Could you check a few things on this model? Use its own coordinates, in mm. A direction names the side the tool comes from. Coordinates: 2 decimals unless noted, no trailing zeros. Write each loop counter-clockwise with the first axis right and the second up, starting at its lowest first coordinate (ties: lowest second). Pieces come first, ordered by that corner, then holes.
```python
from build123d import *

# Parameters (mm, degrees)
SKETCH_1_W          = 95
SKETCH_1_H          = 55
EXTRUDE_1_DEPTH     = 5.5
SKETCH_3_W          = 5.5
SKETCH_3_H          = 20
CUT_EXTRUDE_2_DEPTH = 56.161127617
SKETCH_4_W          = 20
SKETCH_4_H          = 5.504098133
SKETCH_4_W_2        = 5
CUT_EXTRUDE_3_DEPTH = 56.161127617


with BuildPart() as part:
    # ｽｹｯﾁ1 → ﾎﾞｽ - 押し出し1 (new body)
    with BuildSketch(Plane.XY):
        Rectangle(SKETCH_1_W, SKETCH_1_H)
    extrude(amount=EXTRUDE_1_DEPTH)

    # ｽｹｯﾁ3 → ｶｯﾄ - 押し出し2 (cut, through all)
    with BuildSketch(Plane.XY.offset(5.5)):
        with Locations((-44.75, -32)):
            Rectangle(SKETCH_3_W, SKETCH_3_H)
        with Locations((-44.75, 8)):
            Rectangle(SKETCH_3_W, SKETCH_3_H)
    extrude(amount=-CUT_EXTRUDE_2_DEPTH, mode=Mode.SUBTRACT)

    # ｽｹｯﾁ4 → ｶｯﾄ - 押し出し3 (cut, through all)
    with BuildSketch(Plane.XY.offset(5.5)):
        with Locations((-17.5, -24.747950934)):
            Rectangle(SKETCH_4_W, SKETCH_4_H)
        with Locations((22.5, -24.747950934)):
            Rectangle(SKETCH_4_W, SKETCH_4_H)
        with Locations((45, -24.747950934)):
            Rectangle(SKETCH_4_W_2, SKETCH_4_H)
    extrude(amount=-CUT_EXTRUDE_3_DEPTH, mode=Mode.SUBTRACT)


solid = part.part
```
1. For pin 1 (1.5 mm diameter, centred on y = 15.5, z = 3.5, fed in from -X); pin 2 (3 mm diameter, centred on x = 19, z = 3.5, fed in from -Y), each with a flat end and sliding along its axis, tell me the tip position at first contact or that it passes through.
Verdict:
pin 1: stops at x = -42
pin 2: stops at y = -22
2. I want a section at B-B on x = -21. Please give me the cut outline in (y, z), plus the area to 3 significant figures.
Verdict:
outline: (-22, 0) - (27.5, 0) - (27.5, 5.5) - (-22, 5.5) - close
area: 272 mm2
3. I want a section at C-C on y = 4. Please give me the cut outline in (x, z), plus the area to 3 significant figures.
Verdict:
outline: (-42, 0) - (47.5, 0) - (47.5, 5.5) - (-42, 5.5) - close
area: 492 mm2
4. I want a section at A-A on z = 4.15. Please give me the cut outline in (x, y), plus the area to 3 significant figures.
Verdict:
outline: (-47.5, -22) - (-42, -22) - (-42, -27.5) - (-27.5, -27.5) - (-27.5, -22) - (-7.5, -22) - (-7.5, -27.5) - (12.5, -27.5) - (12.5, -22) - (32.5, -22) - (32.5, -27.5) - (42.5, -27.5) - (42.5, -22) - (47.5, -22) - (47.5, 27.5) - (-47.5, 27.5) - (-47.5, 18) - (-42, 18) - (-42, -2) - (-47.5, -2) - close
area: 4,840 mm2
5. If we mould it in two halves opening along X, with no side actions, what happens to faces 1 (the face through (22, -21.996, 3)), 2 (the face through (42.5, -25, 3)), 3 (the face through (-45, 18, 3))? For each: pulls with the +X half, pulls with the -X half, needs draft (parallel to the pull), parting line crosses it, or undercut.
Verdict:
face 1: undercut
face 2: pulls with the +X half
face 3: needs draft
6. On a 3-axis mill with a long thin cutter (end or side, diameter ignored), from which of +Z, -Z, +X, -X, +Y, -Y can I reach the whole of each face in a straight line? I mean faces 4 (the face through (45, -21.996, 3)), 5 (the face through (-42, -25, 3)), 6 (the face through (32.5, -25, 3)). Say none if no direction works.
Verdict:
face 4: +Z, -Z, +X, -Y
face 5: +Z, -Z, -X, -Y
face 6: +Z, -Z, -Y
7. Please list where these lines run through material, in increasing order: line 1 along X through (y, z) = (-22.5, 3.25); line 2 along X through (y, z) = (17.5, 3.2); line 3 along Y through (x, z) = (17.5, 4.8).
Verdict:
line 1: x = -42 to -27.5, -7.5 to 12.5, 32.5 to 42.5
line 2: x = -42 to 47.5
line 3: y = -22 to 27.5
